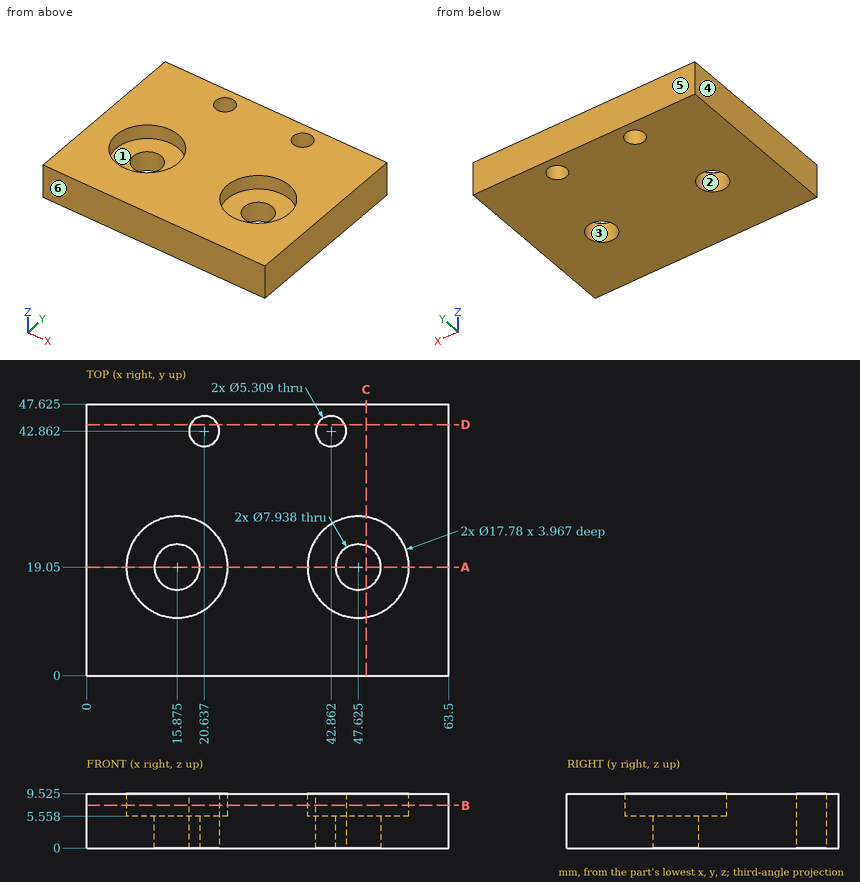
Could you check a few things on this drawing? It's one solid part, dimensions in mm from its lowest x, y, z. A direction names the side the tool comes from. Give positions to 0.01 mm unless a question says otherwise; leave off trailing zeros. Write each loop counter-clockwise with the first axis right and the second up, starting at its lowest first coordinate (ties: lowest second). Pieces come first, ordered by that corner, then holes.
(1) Imagine slicing it at C-C, the plane x = 49. Write out the boundary of the cut face in (y, z) (1 decimal).
Output values:
outline: (0, 0) - (15.3, 0) - (15.3, 5.6) - (10.3, 5.6) - (10.3, 9.5) - (0, 9.5) - close; (22.8, 0) - (47.6, 0) - (47.6, 9.5) - (27.8, 9.5) - (27.8, 5.6) - (22.8, 5.6) - close
(2) If I drill on L1, parallel to X at y = 19.05, z = 3.7; L2, parallel to X at y = 19, z = 9.25 (1 decimal); L3, parallel to Y at x = 22.5, z = 5 (1 decimal), over which ranges is the centre line in solid material (lowest first)?
Output values:
L1: x = 0 to 11.91, 19.84 to 43.66, 51.59 to 63.5
L2: x = 0 to 7, 24.8 to 38.7, 56.5 to 63.5
L3: y = 0 to 41, 44.8 to 47.6
(3) Will this pin go through, and if not, where does the flat tip stop? pin 1 (5.5 mm diameter, centred on x = 17.5, y = 23, fed in from +Z).
Output values:
pin 1: stops at z = 5.56
(4) Thinking about a two-plate mould opening in Y: for the marked faces 3, 4, 5 and 6, which applies, pulls with the +Y half, pulls with the -Y half, needs draft (parallel to the pull), parting line crosses it, or undercut?
Output values:
face 3: undercut
face 4: needs draft
face 5: pulls with the +Y half
face 6: pulls with the -Y half
(5) Imagine slicing it at D-D, the plane y = 44. Write out the boundary of the cut face in (x, z) (1 decimal).
Output values:
outline: (0, 0) - (18.2, 0) - (18.2, 9.5) - (0, 9.5) - close; (23, 0) - (40.5, 0) - (40.5, 9.5) - (23, 9.5) - close; (45.3, 0) - (63.5, 0) - (63.5, 9.5) - (45.3, 9.5) - close
(6) Imagine slicing it at B-B, the plane z = 7.5. Count the separate pieces of the cut face and the enclosed holes in it, and give its area (3 significant figures).
Output values:
separate pieces: 1
enclosed holes: 4
area: 2,480 mm2
(7) Imagine slicing it at A-A, the plane y = 19.05. Write out the boundary of the cut face in (x, z) (1 decimal).
Output values:
outline: (0, 0) - (11.9, 0) - (11.9, 5.6) - (7, 5.6) - (7, 9.5) - (0, 9.5) - close; (19.8, 0) - (43.7, 0) - (43.7, 5.6) - (38.7, 5.6) - (38.7, 9.5) - (24.8, 9.5) - (24.8, 5.6) - (19.8, 5.6) - close; (51.6, 0) - (63.5, 0) - (63.5, 9.5) - (56.5, 9.5) - (56.5, 5.6) - (51.6, 5.6) - close
(8) On a 3-axis mill with a long thin cutter (end or side, diameter ignored), from which of +Z, -Z, +X, -X, +Y, -Y can I reach the whole of each face in a straight line? I mean the marked faces 1 and 2. Say none if no direction works.
Output values:
face 1: +Z
face 2: +Z, -Z
